from build123d import *
from OCP.BRepFilletAPI import BRepFilletAPI_MakeChamfer

# Parameters (mm, degrees)
SKETCH1_W           = 40
SKETCH1_H           = 40
BOSS_EXTRUDE1_DEPTH = 4
CUT_EXTRUDE1_REACH  = 30.566
SKETCH2_R           = 2.75
BOSS_EXTRUDE2_DEPTH = 8
CHAMFER1_SIZE       = 10
CHAMFER1_SIZE2      = 11.917535926
SKETCH4_R           = 2.75
CUT_EXTRUDE2_DEPTH  = 7
BOSS_EXTRUDE3_DEPTH = 2.75
CHAMFER2_SIZE       = 1.5
FILLET1_R           = 5
CHAMFER3_SIZE       = 2


with BuildPart() as part:
    # Sketch1 → Boss-Extrude1 (new body)
    with BuildSketch(Plane.XY):
        Rectangle(SKETCH1_W, SKETCH1_H)
    extrude(amount=BOSS_EXTRUDE1_DEPTH)

    # Sketch2 → Cut-Extrude1 (cut, up to next)
    with BuildSketch(Plane.XY, mode=Mode.PRIVATE) as cut_extrude1_sk1:
        with Locations((-13, 13)):
            Circle(SKETCH2_R)
    cut_extrude1_tool1 = extrude(cut_extrude1_sk1.sketch, amount=CUT_EXTRUDE1_REACH, mode=Mode.PRIVATE) & part.part
    # Sketch2 → Cut-Extrude1 (cut, up to next)
    with BuildSketch(Plane.XY, mode=Mode.PRIVATE) as cut_extrude1_sk2:
        with Locations(Location((13, 13, 0), (0, 0, 180))):
            Circle(SKETCH2_R)
    cut_extrude1_tool2 = extrude(cut_extrude1_sk2.sketch, amount=CUT_EXTRUDE1_REACH, mode=Mode.PRIVATE) & part.part
    # Sketch2 → Cut-Extrude1 (cut, up to next)
    with BuildSketch(Plane.XY, mode=Mode.PRIVATE) as cut_extrude1_sk3:
        with Locations((13, -13)):
            Circle(SKETCH2_R)
    cut_extrude1_tool3 = extrude(cut_extrude1_sk3.sketch, amount=CUT_EXTRUDE1_REACH, mode=Mode.PRIVATE) & part.part
    # Sketch2 → Cut-Extrude1 (cut, up to next)
    with BuildSketch(Plane.XY, mode=Mode.PRIVATE) as cut_extrude1_sk4:
        with Locations(Location((-13, -13, 0), (0, 0, 180))):
            Circle(SKETCH2_R)
    cut_extrude1_tool4 = extrude(cut_extrude1_sk4.sketch, amount=CUT_EXTRUDE1_REACH, mode=Mode.PRIVATE) & part.part
    add(cut_extrude1_tool1.solids().sort_by_distance((-13, 13, 0))[0], mode=Mode.SUBTRACT)
    add(cut_extrude1_tool2.solids().sort_by_distance((13, 13, 0))[0], mode=Mode.SUBTRACT)
    add(cut_extrude1_tool3.solids().sort_by_distance((13, -13, 0))[0], mode=Mode.SUBTRACT)
    add(cut_extrude1_tool4.solids().sort_by_distance((-13, -13, 0))[0], mode=Mode.SUBTRACT)

    # Sketch3 → Boss-Extrude2 (add, symmetric)
    with BuildSketch(Plane(origin=(0, 0, 0), x_dir=(1, 0, 0), z_dir=(0, 1, 0))):
        with BuildLine():
            Line((-7, -4), (-7, -42))
            Line((-7, -42), (3, -42))
            Line((3, -42), (3, -32.261355821))
            ThreePointArc((3, -32.261355821), (-3.261355821, -22), (7, -15.738644179))
            Line((7, -15.738644179), (7, -4))
            Line((7, -4), (-7, -4))
        make_face()
    extrude(amount=BOSS_EXTRUDE2_DEPTH, both=True)

    # Chamfer1: one chamfer whose edges measure the first distance from different faces: ONE call of the kernel's chamfer builder (chamfer() names one face for all edges)
    chamfer1_edges_1 = [part.edges().sort_by_distance(p)[0] for p in [
        (0, -8, 4),
    ]]
    chamfer1_side_1 = [part.faces().sort_by_distance(p)[0] for p in [
        (6.595030865, -8, 9.86932209),
    ]]
    chamfer1_edges_2 = [part.edges().sort_by_distance(p)[0] for p in [
        (0, 8, 4),
    ]]
    chamfer1_side_2 = [part.faces().sort_by_distance(p)[0] for p in [
        (6.595030865, 8, 9.86932209),
    ]]
    chamfer1 = BRepFilletAPI_MakeChamfer(part.part.solid().wrapped)
    for e in chamfer1_edges_1:
        chamfer1.Add(CHAMFER1_SIZE, CHAMFER1_SIZE2, e.wrapped, chamfer1_side_1[0].wrapped)  # the first distance lies on this face
    for e in chamfer1_edges_2:
        chamfer1.Add(CHAMFER1_SIZE, CHAMFER1_SIZE2, e.wrapped, chamfer1_side_2[0].wrapped)  # the first distance lies on this face
    add(Compound.cast(chamfer1.Shape()), mode=Mode.REPLACE)

    # Sketch4 → Cut-Extrude2 (cut, symmetric)
    with BuildSketch(Plane(origin=(0, 0, 0), x_dir=(0, 0, -1), z_dir=(1, 0, 0))):
        with Locations((-12, 0)):
            Circle(SKETCH4_R)
        with Locations((-36, 0)):
            Circle(SKETCH4_R)
    extrude(amount=CUT_EXTRUDE2_DEPTH, both=True, mode=Mode.SUBTRACT)

    # Sketch5 → Boss-Extrude3 (add, symmetric)
    with BuildSketch(Plane(origin=(0, 0, 0), x_dir=(1, 0, 0), z_dir=(0, 1, 0))):
        with BuildLine():
            Line((7, -15.738644179), (7, -18.184288522))
            ThreePointArc((7, -18.184288522), (-0.815711478, -22), (3, -29.815711478))
            Line((3, -29.815711478), (3, -32.261355821))
            ThreePointArc((3, -32.261355821), (-3.261355821, -22), (7, -15.738644179))
        make_face()
    extrude(amount=BOSS_EXTRUDE3_DEPTH, both=True)

    # Chamfer2
    chamfer2_edges = [part.edges().sort_by_distance(p)[0] for p in [
        (7, 0, 4),
        (-7, 0, 4),
    ]]
    chamfer(chamfer2_edges, length=CHAMFER2_SIZE)

    # Fillet1
    fillet1_edges = [part.edges().sort_by_distance(p)[0] for p in [
        (20, -20, 2),
        (-20, -20, 2),
        (-20, 20, 2),
        (20, 20, 2),
    ]]
    fillet(fillet1_edges, radius=FILLET1_R)

    # Chamfer3
    chamfer3_edges = [part.edges().sort_by_distance(p)[0] for p in [
        (-7, -8, 28),
        (-7, 8, 28),
    ]]
    chamfer(chamfer3_edges, length=CHAMFER3_SIZE)


solid = part.part
Work out the finished part from the listing and answer in its coordinate system (mm). A direction names the side the tool comes from. Coordinates: 2 decimals unless noted, no trailing zeros. Write each loop counter-clockwise with the first axis right and the second up, starting at its lowest first coordinate (ties: lowest second). Pieces come first, ordered by that corner, then holes. Notation, with made-up numbers: M -7,-36 L 1,-36 A30 cw 1,-6 Z; hole C -27,62 d11. An arc over 180 degrees is marked long. Write item = value, one per line.
1. The part is cut by section B-B (z = 36). Determine the outline of the cut face in (x, y), then the cut area to 3 significant figures.
Solution:
outline = M -7,-6 L -5,-8 L 3,-8 L 3,-2.75 L -7,-2.75 Z; M -7,2.75 L 3,2.75 L 3,8 L -5,8 L -7,6 Z
area = 101 mm2
2. For faces 5 (the face through (7, 0, 9)), 6 (the face through (-7.7, -0.3, 4.8)), 7 (the face through (-6, -7, 28)), determine the directions among +Z, -Z, +X, -X, +Y, -Y from which every point of the face is accessible in a straight line to the end or side of a thin tool.
Solution:
face_5 = +Z, +X, +Y, -Y
face_6 = +Z, -X, +Y, -Y
face_7 = +Z, -X, -Y
3. Determine the mould class of faces 1 (the face through (-2, 0, 42)), 2 (the face through (-0.1, -1.05, 9.46)), 3 (the face through (-18, -19, 2)), 4 (the face through (-1, 2.75, 21)) for opening direction Z: released by +Z, released by -Z, zero draft, split by the parting line, or undercut.
Solution:
face_1 = released by +Z
face_2 = undercut
face_3 = zero draft
face_4 = undercut
4. The part is cut by section A-A (y = 0). Determine the outline of the cut face in (x, z).
Solution:
outline = M -20,0 L 20,0 L 20,4 L 8.5,4 L 7,5.5 L 7,9.25 L -7,9.25 L -7,5.5 L -8.5,4 L -20,4 Z; M -7,14.75 L 7,14.75 L 7,18.18 A6.15 cw 3,29.82 L 3,33.25 L -7,33.25 Z; M -7,38.75 L 3,38.75 L 3,42 L -7,42 Z
5. Straight lines are drawn through the part: line 1 (Y direction, x = 13, z = 1.55); line 2 (Y direction, x = 0, z = 36). For each, find the intervals that lie inside material, in ascending order. Write a range as from..to.
Solution:
line_1 = -20..-15.75, -10.25..10.25, 15.75..20
line_2 = -8..-2.75, 2.75..8
6. The part is cut by section C-C (x = 13). Determine the outline of the cut face in (y, z), then the cut area to 3 significant figures.
Solution:
outline = M -20,0 L -15.75,0 L -15.75,4 L -20,4 Z; M -10.25,0 L 10.25,0 L 10.25,4 L -10.25,4 Z; M 15.75,0 L 20,0 L 20,4 L 15.75,4 Z
area = 116 mm2
7. The part is cut by section D-D (y = -7). Determine the outline of the cut face in (x, z), then the cut area to 3 significant figures.
Solution:
outline = M -20,0 L 20,0 L 20,4 L 8.5,4 L 7,5.5 L 7,15.74 A8.5 cw 3,32.26 L 3,42 L -6,42 L -6,14.84 L -7,14.84 L -7,5.5 L -8.5,4 L -20,4 Z
area = 482 mm2
8. Flat-ended cylindrical pins translate along their axes: pin 1 (6.5 mm diameter, centred on x = 13, y = 13, fed in from +Z); pin 2 (12 mm diameter, centred on x = -7, z = 20.5, fed in from +Y); pin 3 (8 mm diameter, centred on y = 13, z = 10.5, fed in from +X); pin 4 (8 mm diameter, centred on x = -3, y = -11, fed in from +Z). Find the tip coordinate at first contact, or state that the pin passes through.
Solution:
pin_1 = 4
pin_2 = 8
pin_3 = 7
pin_4 = 42
